Input: dimensioned drawing with shaded views. Units: mm. Origin: part minimum x, y, z. A direction names the side the tool comes from. Round coordinates to 2 decimals unless told otherwise and drop trailing zeros. Write each loop counter-clockwise with the first axis right and the second up, starting at its lowest first coordinate (ties: lowest second). Pieces come first, ordered by that corner, then holes. Notation, with made-up numbers: (2, -0.75) -> (8, -0.75) arc R17 cw to (8, 6.25) -> close; hole circle Ø7 at (71.5, -36). An arc over 180 degrees is marked (long way). One line per item, written item: value. Start each with the question number.
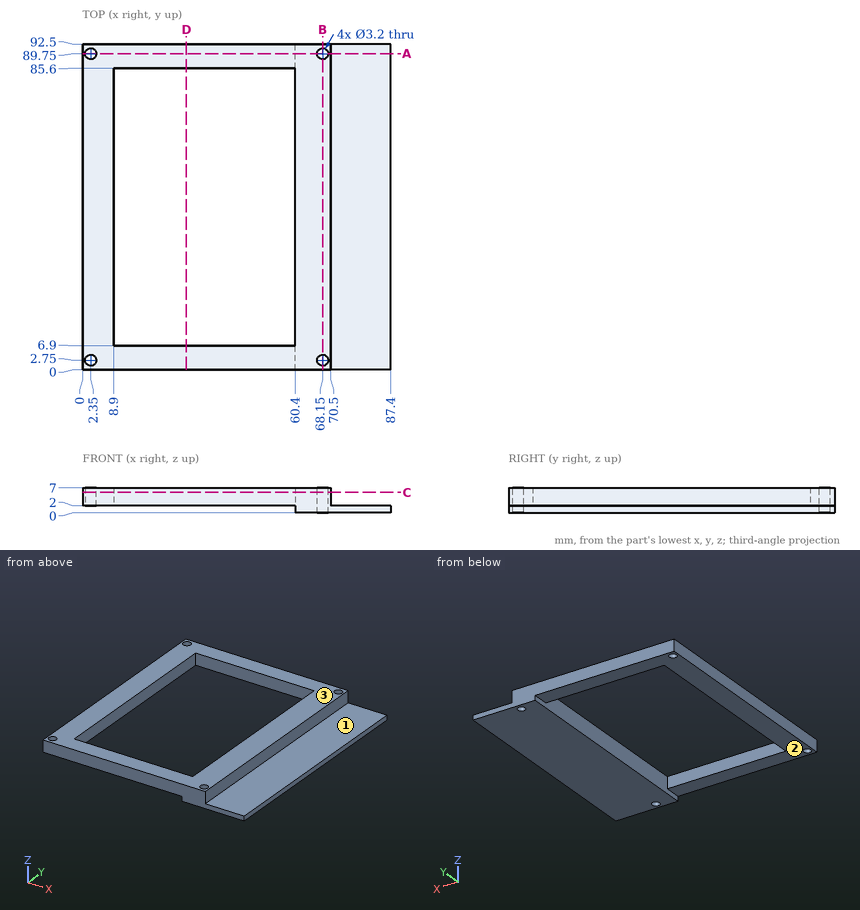
(1) Section query D-D (x = 29.5). Output: boundary loops of the cut face in (y, z).
(2) Line query: probe 1 along Y at (x, z) = (68.15, 4.5); probe 2 along Y at (x, z) = (27, 4.5); probe 3 along X at (y, z) = (21, 3.5). Output: solid intervals per line, ascending.
(3) Set-up query: the marked faces 1, 2 and 3. Return all of +Z, -Z, +X, -X, +Y, -Y with unobstructed straight access to the full face (end or side cutting, diameter ignored); none if empty.
(4) Section query B-B (x = 68.15). Output: boundary loops of the cut face in (y, z), and give its area (3 significant figures).
(5) Pin query (flat end, axial travel): pin 1 (1.9 mm diameter, centred on x = 68.15, y = 89.75, fed in from +Z); pin 2 (5 mm diameter, centred on x = 77.5, y = 25.5, fed in from +Z); pin 3 (4 mm diameter, centred on y = 56.5, z = 5, fed in from +X); pin 4 (3.5 mm diameter, centred on x = 2.35, y = 2.75, fed in from -Z). Return the tip coordinate at first contact, or that it passes through.
(6) Section query A-A (y = 89.75). Output: boundary loops of the cut face in (x, z), and give its area (3 significant figures).
(7) Section query C-C (z = 5.75). Output: boundary loops of the cut face in (x, y), and give its area (3 significant figures).
Results list:
1. outline: (0, 2) -> (6.9, 2) -> (6.9, 7) -> (0, 7) -> close; (85.6, 2) -> (92.5, 2) -> (92.5, 7) -> (85.6, 7) -> close
2. probe 1: y = 0 to 1.15, 4.35 to 88.15, 91.35 to 92.5
2. probe 2: y = 0 to 6.9, 85.6 to 92.5
2. probe 3: x = 0 to 8.9, 60.4 to 70.5
3. face 1: +Z, +X, +Y, -Y
3. face 2: -Z, -X, +Y, -Y
3. face 3: +Z, +X, -X, +Y, -Y
4. outline: (0, 0) -> (1.15, 0) -> (1.15, 7) -> (0, 7) -> close; (4.35, 0) -> (88.15, 0) -> (88.15, 7) -> (4.35, 7) -> close; (91.35, 0) -> (92.5, 0) -> (92.5, 7) -> (91.35, 7) -> close
4. area: 603 mm^2
5. pin 1: passes through
5. pin 2: stops at z = 2
5. pin 3: stops at x = 70.5
5. pin 4: stops at z = 2
6. outline: (0, 2) -> (0.75, 2) -> (0.75, 7) -> (0, 7) -> close; (3.95, 2) -> (60.4, 2) -> (60.4, 0) -> (66.55, 0) -> (66.55, 7) -> (3.95, 7) -> close; (69.75, 0) -> (87.4, 0) -> (87.4, 2) -> (70.5, 2) -> (70.5, 7) -> (69.75, 7) -> close
6. area: 368 mm^2
7. outline: (0, 0) -> (70.5, 0) -> (70.5, 92.5) -> (0, 92.5) -> close; hole circle Ø3.2 at (2.35, 2.75); hole circle Ø3.2 at (2.35, 89.75); hole (8.9, 6.9) -> (60.4, 6.9) -> (60.4, 85.6) -> (8.9, 85.6) -> close; hole circle Ø3.2 at (68.15, 2.75); hole circle Ø3.2 at (68.15, 89.75)
7. area: 2,440 mm^2
